Autodesk Inventor part; units mm, degrees
ref_plane "YZ Plane" through (0, 0, 0) normal (1, 0, 0) x (0, 1, 0)
ref_plane "XZ Plane" through (0, 0, 0) normal (0, 1, 0) x (-1, 0, 0)
ref_plane "XY Plane" through (0, 0, 0) normal (0, 0, 1) x (1, 0, 0)
sketch "Sketch1" plane through (0, 0, 0) normal (0, 1, 0) x (-1, 0, 0)
  line L0 (0, 0) -> (-70, 0)
  line L1 (-70, 0) -> (-70, -30)
  line L2 (-70, -30) -> (0, -30)
  line L3 (0, -30) -> (0, 0)
  circle A0 centre (-5.75, -3.5) radius 1.5
  circle A1 centre (-5.75, -26.5) radius 1.5
  circle A2 centre (-64.25, -3.5) radius 1.5
  circle A3 centre (-64.25, -26.5) radius 1.5
  line L4 (-5.75, -3.5) -> (-5.75, -26.5) construction
  line L5 (-5.75, -26.5) -> (-64.25, -26.5) construction
  line L6 (-64.25, -26.5) -> (-64.25, -3.5) construction
  line L7 (-64.25, -3.5) -> (-5.75, -3.5) construction
  dimension "d0" = 70
  dimension "d1" = 30
  dimension "d2" = 3
  dimension "d3" = 3
  dimension "d4" = 3
  dimension "d5" = 3
  dimension "d6" = 55.5
  dimension "d8" = 20
  dimension "d10" = 4.25
  dimension "d11" = 4.25
  dimension "d12" = 3.5
  dimension "d13" = 3.5
extrude "Extrusion1" add sketch "Sketch1" along normal blind 1.5
sketch "Sketch2" plane through (0, 0, 0) normal (0, -1, 0) x (1, 0, 0)
  line L0 (12.3126, -6.7897) -> (54.4692, -6.7897)
  line L1 (54.4692, -6.7897) -> (54.4692, -21.3823)
  line L2 (54.4692, -21.3823) -> (12.3126, -21.3823)
  line L3 (12.3126, -21.3823) -> (12.3126, -6.7897)
  point P0 (0, 0)
extrude "Extrusion2" add sketch "Sketch2" along normal blind 7.5
equation "\"d10\" = d11"
equation "\"d12\" = d13"
properties part number "my_own_pcb"
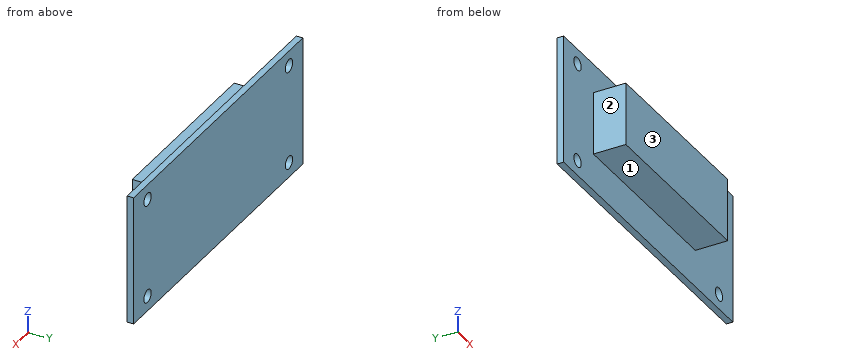
The model under review builds one solid part; all positions refer to its coordinate system, in mm. Face numbers are marked on the shaded views. A direction names the side the tool comes from. Give positions to 0.01 mm unless a question says otherwise; leave off trailing zeros. Write each loop counter-clockwise with the first axis right and the second up, starting at its lowest first coordinate (ties: lowest second). Pieces come first, ordered by that corner, then holes.
1. Add section A-A, the plane x = 64.25. Write out the cut boundary in (y, z).
2. Tool access review of the marked faces 1, 2 and 3: name each direction out of +Z, -Z, +X, -X, +Y, -Y from which nothing blocks a thin tool from reaching the whole face with its end or side.
3. Add section B-B, the plane z = -26.5. Write out the cut boundary in (x, y).
4. Add section C-C, the plane z = -10.5. Write out the cut boundary in (x, y).
5. For P1, Ø1, axis at x = 51, z = -23.5, coming from the -Y side; P2, Ø2, axis at x = 30.5, y = -3.5, coming from the -Z side; P3, Ø4, axis at x = 34.5, y = -5.5, coming from the +Z side; P4, Ø2.5, axis at x = 5.75, z = -3.5, coming from the -Y side, all flat-tipped, find the tip position at first contact; note any pin that passes through.
6. Wall thickness on L1, parallel to Z at x = 64.25, y = 0.3; L2, parallel to Y at x = 11, z = -19.5; L3, parallel to X at y = 1, z = -2.5: over which ranges is each line inside the solid? List them lowest first.
7. Add section D-D, the plane x = 52. Write out the cut boundary in (y, z), plus the area to 3 significant figures.
Worked answers:
1. outline: (0, -30) - (1.5, -30) - (1.5, -28) - (0, -28) - close; (0, -25) - (1.5, -25) - (1.5, -5) - (0, -5) - close; (0, -2) - (1.5, -2) - (1.5, 0) - (0, 0) - close
2. face 1: -Z, +X, -X, -Y
2. face 2: +Z, -Z, -X, -Y
2. face 3: +Z, -Z, +X, -X, -Y
3. outline: (0, 0) - (4.25, 0) - (4.25, 1.5) - (0, 1.5) - close; (7.25, 0) - (62.75, 0) - (62.75, 1.5) - (7.25, 1.5) - close; (65.75, 0) - (70, 0) - (70, 1.5) - (65.75, 1.5) - close
4. outline: (0, 0) - (12.31, 0) - (12.31, -7.5) - (54.47, -7.5) - (54.47, 0) - (70, 0) - (70, 1.5) - (0, 1.5) - close
5. P1: stops at y = 0
5. P2: stops at z = -21.38
5. P3: stops at z = -6.79
5. P4: passes through
6. L1: z = -30 to -28, -25 to -5, -2 to 0
6. L2: y = 0 to 1.5
6. L3: x = 0 to 4.63, 6.87 to 63.13, 65.37 to 70
7. outline: (-7.5, -21.38) - (0, -21.38) - (0, -30) - (1.5, -30) - (1.5, 0) - (0, 0) - (0, -6.79) - (-7.5, -6.79) - close
7. area: 154 mm2
